Autodesk Inventor part; units mm, degrees
ref_plane "YZ Plane" through (0, 0, 0) normal (1, 0, 0) x (0, 1, 0)
ref_plane "XZ Plane" through (0, 0, 0) normal (0, 1, 0) x (-1, 0, 0)
ref_plane "XY Plane" through (0, 0, 0) normal (0, 0, 1) x (1, 0, 0)
sketch "Sketch1" plane through (0, 0, 0) normal (0, 1, 0) x (-1, 0, 0)
  line L0 (-6.35, -3.6662) -> (-6.35, 3.6662)
  line L1 (-6.35, 3.6662) -> (0, 7.3323)
  line L2 (0, 7.3323) -> (6.35, 3.6662)
  line L3 (6.35, 3.6662) -> (6.35, -3.6662)
  line L4 (6.35, -3.6662) -> (0, -7.3323)
  line L5 (0, -7.3323) -> (-6.35, -3.6662)
  point P0 (0, 0)
  point P1 (0, 0)
  dimension "d0" = 12.7
extrude "Extrusion1" add sketch "Sketch1" along normal blind 130.175
sketch "Sketch3" plane through (0, 130.175, 0) normal (0, 1, 0) x (1, 0, 0)
  circle A0 centre (0, 0) radius 2.5527
  dimension "d3" = 5.1054
extrude "Extrusion2" cut sketch "Sketch3" against normal blind 25.4
sketch "Sketch4" plane through (0, 0, 0) normal (0, -1, 0) x (1, 0, 0)
  circle A0 centre (0, 0) radius 2.5527
  dimension "d6" = 5.1054
extrude "Extrusion3" cut sketch "Sketch4" against normal blind 25.4
properties part number "INDX_017_Mainhex" material "Aluminum 6061"
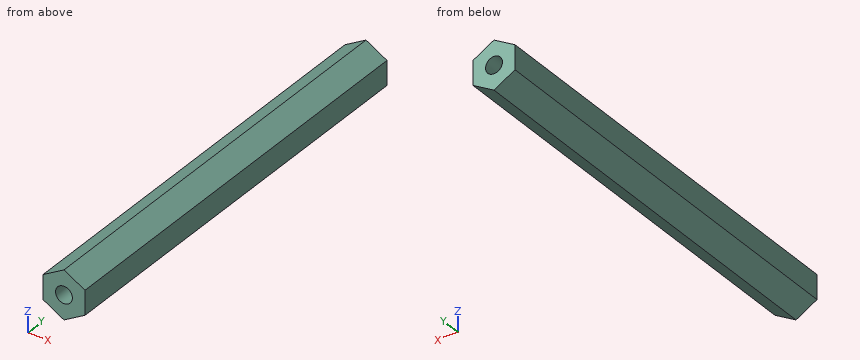
Build history of the part. All positions in model axes, mm. Give positions to 0.01 mm unless a question says otherwise; leave off trailing zeros. Order: outer loops, then holes, each group sorted by start corner. A loop starts at its lowest first (then second) coordinate and runs counter-clockwise, first axis right, second up. Notation, with made-up numbers: M 0,-22.5 L 44,-22.5 A32 ccw 44,12.5 Z; hole C 77,8 d3. An arc over 180 degrees is marked long. Put each result on its own line as item: value.
Item 1: Drop flat-ended pins along their axis: pin 1 Ø6 at (x, y) = (0, 99) entering from +Z; pin 2 Ø4 at (x, y) = (4.5, 105) entering from +Z; pin 3 Ø4 at (x, z) = (0, 0) entering from +Y (3 decimals). Give the stop position or say it passes through.
Results are:
pin 1: z = 7.33
pin 2: z = 5.89
pin 3: y = 104.775
Item 2: Cut at C-C on x = 4.75. Write the cut outline in (y, z) (3 decimals), then the cut area to 3 significant figures.
Results are:
outline: M 0,-4.59 L 130.175,-4.59 L 130.175,4.59 L 0,4.59 Z
area: 1,190 mm2
Item 3: Cut at A-A on z = 0. Write the cut outline in (x, y) (3 decimals).
Results are:
outline: M -6.35,0 L -2.553,0 L -2.553,25.4 L 2.553,25.4 L 2.553,0 L 6.35,0 L 6.35,130.175 L 2.553,130.175 L 2.553,104.775 L -2.553,104.775 L -2.553,130.175 L -6.35,130.175 Z
Item 4: Cut at B-B on y = 95. Write the cut outline in (x, z), then the cut area to 3 significant figures.
Results are:
outline: M -6.35,-3.67 L 0,-7.33 L 6.35,-3.67 L 6.35,3.67 L 0,7.33 L -6.35,3.67 Z
area: 140 mm2
Item 5: Wall check: probe 1 along X at (y, z) = (124.5, 0.25); probe 2 along Z at (x, y) = (0, 14); probe 3 along Y at (x, z) = (1.5, -1.5) (3 decimals). Give the ranges that are in metal, low to high.
Results are:
probe 1: -6.35 to -2.54, 2.54 to 6.35
probe 2: -7.33 to -2.55, 2.55 to 7.33
probe 3: 25.4 to 104.775
